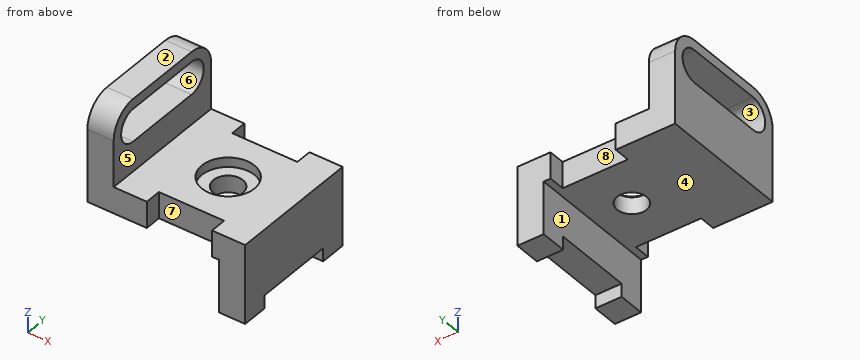
```python
from build123d import *

# Parameters (mm, degrees)
F0_W     = 31.496
F0_H     = 12.7
F1_DEPTH = 23.876
F2_DEPTH = 31.75
F3_W     = 38.1
F3_H     = 6.35
F4_DEPTH = 76.201
F6_DEPTH = 25.4
F7_R     = 7.112
F8_DEPTH = 38.101
F7_R_2   = 12.7
F9_DEPTH = 4.572


with BuildPart() as f1:
    # F0 (on Front) → F1 (new body, symmetric)
    with BuildSketch(Plane.XZ):
        with Locations((44.45, 6.35)):
            Rectangle(F0_W, F0_H)
    extrude(amount=F1_DEPTH, both=True)

    # F0 (on Front) → F2 (join, symmetric)
    with BuildSketch(Plane.XZ):
        Polygon((0, 47.752), (0, 0), (28.702, 0), (28.702, 12.7), (12.7, 12.7), (12.7, 47.752), align=None)
        Polygon((60.198, 12.7), (60.198, 0), (63.5, 0), (63.5, -25.4), (76.2, -25.4), (76.2, 12.7), align=None)
    extrude(amount=F2_DEPTH, both=True)

    # F3 (on face) → F4 (cut, through all)
    with BuildSketch(Plane.YZ.offset(76.2)):
        with Locations((0, -22.225)):
            Rectangle(F3_W, F3_H)
    extrude(amount=-F4_DEPTH, mode=Mode.SUBTRACT)

    # F5 (on face) → F6 (cut)
    with BuildSketch(Plane.YZ.offset(12.7)):
        with BuildLine():
            ThreePointArc((-31.75, 35.052), (-28.030256, 44.032256), (-19.05, 47.752))
            Line((-19.05, 47.752), (-31.75, 47.752))
            Line((-31.75, 47.752), (-31.75, 35.052))
        make_face()
        with BuildLine():
            Line((19.05, 42.926), (-19.05, 42.926))
            ThreePointArc((-19.05, 42.926), (-26.924, 35.052), (-19.05, 27.178))
            Line((-19.05, 27.178), (19.05, 27.178))
            ThreePointArc((19.05, 27.178), (26.924, 35.052), (19.05, 42.926))
        make_face()
        with BuildLine():
            Line((31.75, 47.752), (19.05, 47.752))
            ThreePointArc((19.05, 47.752), (28.030256, 44.032256), (31.75, 35.052))
            Line((31.75, 35.052), (31.75, 47.752))
        make_face()
    extrude(amount=-F6_DEPTH, mode=Mode.SUBTRACT)

    # F7 (on face) → F8 (cut, through all)
    with BuildSketch(Plane.XY.offset(12.7)):
        with Locations((44.45, 0)):
            Circle(F7_R)
    extrude(amount=-F8_DEPTH, mode=Mode.SUBTRACT)

    # F7 (on face) → F9 (cut)
    with BuildSketch(Plane.XY.offset(12.7)):
        with Locations((44.45, 0)):
            Circle(F7_R_2)
        with Locations((44.45, 0)):
            Circle(F7_R, mode=Mode.SUBTRACT)
    extrude(amount=-F9_DEPTH, mode=Mode.SUBTRACT)


solid = f1.part
```
Build history of the part. All positions in model axes, mm. Face numbers are marked on the shaded views. A direction names the side the tool comes from. Give positions to 0.01 mm unless a question says otherwise; leave off trailing zeros. Loops run counter-clockwise (first coordinate to the right, second up) from the corner with the lowest first, then second, coordinate; pieces in that order, holes last. Notation, with made-up numbers: (27.25, 75.5) -> (77.25, 75.5) arc R27 ccw to (77.25, 93.5) -> close; hole circle Ø1 at (10, 9). An arc over 180 degrees is marked (long way). One line per question, with ' | ' between items.
Q1. Cut at A-A, the plane y = 0. Write the cut outline in (x, z), plus the area to 3 significant figures.
Filled sheet:
outline: (0, 0) -> (37.34, 0) -> (37.34, 8.13) -> (31.75, 8.13) -> (31.75, 12.7) -> (12.7, 12.7) -> (12.7, 27.18) -> (0, 27.18) -> close; (0, 42.93) -> (12.7, 42.93) -> (12.7, 47.75) -> (0, 47.75) -> close; (51.56, 0) -> (63.5, 0) -> (63.5, -19.05) -> (76.2, -19.05) -> (76.2, 12.7) -> (57.15, 12.7) -> (57.15, 8.13) -> (51.56, 8.13) -> close | area: 1,220 mm²
Q2. Cut at B-B, the plane x = 44.45. Write the cut outline in (y, z).
Filled sheet:
outline: (-23.88, 0) -> (-7.11, 0) -> (-7.11, 8.13) -> (-12.7, 8.13) -> (-12.7, 12.7) -> (-23.88, 12.7) -> close; (7.11, 0) -> (23.88, 0) -> (23.88, 12.7) -> (12.7, 12.7) -> (12.7, 8.13) -> (7.11, 8.13) -> close
Q3. Cut at D-D, the plane x = 10.5. Write the cut outline in (y, z).
Filled sheet:
outline: (-31.75, 0) -> (31.75, 0) -> (31.75, 35.05) arc R12.7 ccw to (19.05, 47.75) -> (-19.05, 47.75) arc R12.7 ccw to (-31.75, 35.05) -> close; hole (-19.05, 27.18) -> (19.05, 27.18) arc R7.87 ccw to (19.05, 42.93) -> (-19.05, 42.93) arc R7.87 ccw to start
Q4. Pull direction Z, two halves, no side cores. Call the marked faces 1, 2 and 3: pulls with the +Z half, pulls with the -Z half, needs draft (parallel to the pull), parting line crosses it, or undercut.
Filled sheet:
face 1: needs draft | face 2: pulls with the +Z half | face 3: undercut
Q5. Drop flat-ended pins along their axis: pin 1 (10 mm diameter, centred on x = 60, y = -15, fed in from -Z); pin 2 (3 mm diameter, centred on x = 33.5, y = -15.5, fed in from -Z); pin 3 (14 mm diameter, centred on x = 49.5, z = 6.5, fed in from +Y); pin 4 (5 mm diameter, centred on x = 58, z = 12, fed in from -Y). Give the stop position or say it passes through.
Filled sheet:
pin 1: stops at z = -19.05 | pin 2: stops at z = 0 | pin 3: stops at y = 23.88 | pin 4: stops at y = -31.75
Q6. Cut at C-C, the plane y = 14.5. Write the cut outline in (x, z).
Filled sheet:
outline: (0, 0) -> (63.5, 0) -> (63.5, -19.05) -> (76.2, -19.05) -> (76.2, 12.7) -> (12.7, 12.7) -> (12.7, 27.18) -> (0, 27.18) -> close; (0, 42.93) -> (12.7, 42.93) -> (12.7, 47.75) -> (0, 47.75) -> close
Q7. Drill centre lines: line 1 along Y through (x, z) = (44, 3); line 2 along Y through (x, z) = (68, -20.5); line 3 along Z through (x, y) = (7, -13). Where is each one in solid material? Low to high. Write a range as [from, to].
Filled sheet:
line 1: y = [-23.88, -7.1], [7.1, 23.88] | line 2: y = [-31.75, -19.05], [19.05, 31.75] | line 3: z = [0, 27.18], [42.93, 47.75]
Q8. Tool access for the marked faces 4, 5, 6, 7 and 8: list every direction of +Z, -Z, +X, -X, +Y, -Y with a clear straight run to the whole face (end or side of a thin tool).
Filled sheet:
face 4: -Z, -X, +Y, -Y | face 5: +Z, +X, +Y, -Y | face 6: +X, -X | face 7: +Z, -Z, -Y | face 8: +Z, -Z, +Y
